from build123d import *

# Parameters (mm, degrees)
F0_R         = 8.5
F1_DEPTH     = 16
F2_DEPTH     = 4
F3_DEPTH     = 15
F4_W         = 9.6
F4_H         = 9.6
F5_DEPTH     = 11
F6_T1_DEPTH  = 10
F6_T3_DEPTH  = 7.6
F6_T5_DEPTH  = 7.6
F6_S9_W      = 1.02
F6_S9_H      = 1.02
F6_T10_DEPTH = 1.02
F6_S15_W     = 1.02
F6_S15_H     = 1.02
F6_T16_DEPTH = 1.02
F6_S21_W     = 1.02
F6_S21_H     = 1.02
F6_T22_DEPTH = 1.02
F6_S27_W     = 1.02
F6_S27_H     = 1.02
F6_T28_DEPTH = 1.02
F7_SIZE2     = 25
F7_SIZE      = 1
F8_T1_DEPTH  = 4
F8_T3_DEPTH  = 4
F9_DEPTH     = 25


# Not quite as in the source:
# - a fillet or chamfer that OpenCascade refuses, or shapes differently, is made with other operations: its cross-section is extruded or revolved along the edge and cut away or added


with BuildPart() as f1:
    # F0 (on Top) → F1 (new body)
    with BuildSketch(Plane.XY):
        Circle(F0_R)
        with BuildLine():
            Line((3.4119543857, 2.130107217), (3.5507041555, 2.05))
            Line((3.5507041555, 2.05), (3.5507041555, -2.05))
            Line((3.5507041555, -2.05), (3.4119543857, -2.130107217))
            ThreePointArc((3.4119543857, -2.130107217), (0, -4.85), (-3.4119543857, -2.130107217))
            Line((-3.4119543857, -2.130107217), (-3.5507041555, -2.05))
            Line((-3.5507041555, -2.05), (-3.5507041555, 2.05))
            Line((-3.5507041555, 2.05), (-3.4119543857, 2.130107217))
            ThreePointArc((-3.4119543857, 2.130107217), (0, 4.85), (3.4119543857, 2.130107217))
        make_face(mode=Mode.SUBTRACT)
    extrude(amount=F1_DEPTH)

    # F0 (on Top) → F2 (join)
    with BuildSketch(Plane.XY):
        with BuildLine():
            Line((0, 4.1), (3.4119543857, 2.130107217))
            ThreePointArc((3.4119543857, 2.130107217), (0, 4.85), (-3.4119543857, 2.130107217))
            Line((-3.4119543857, 2.130107217), (0, 4.1))
        make_face()
        with BuildLine():
            ThreePointArc((-3.4119543857, -2.130107217), (0, -4.85), (3.4119543857, -2.130107217))
            Line((3.4119543857, -2.130107217), (0, -4.1))
            Line((0, -4.1), (-3.4119543857, -2.130107217))
        make_face()
    extrude(amount=F2_DEPTH)

    # F0 (on Top) → F3 (join)
    with BuildSketch(Plane.XY):
        Circle(F0_R)
        with BuildLine():
            Line((3.4119543857, 2.130107217), (3.5507041555, 2.05))
            Line((3.5507041555, 2.05), (3.5507041555, -2.05))
            Line((3.5507041555, -2.05), (3.4119543857, -2.130107217))
            ThreePointArc((3.4119543857, -2.130107217), (0, -4.85), (-3.4119543857, -2.130107217))
            Line((-3.4119543857, -2.130107217), (-3.5507041555, -2.05))
            Line((-3.5507041555, -2.05), (-3.5507041555, 2.05))
            Line((-3.5507041555, 2.05), (-3.4119543857, 2.130107217))
            ThreePointArc((-3.4119543857, 2.130107217), (0, 4.85), (3.4119543857, 2.130107217))
        make_face(mode=Mode.SUBTRACT)
        with BuildLine():
            ThreePointArc((-3.5, 1.35), (-3.4779189431, 1.7425300307), (-3.4119543857, 2.130107217))
            Line((-3.4119543857, 2.130107217), (-3.5507041555, 2.05))
            Line((-3.5507041555, 2.05), (-3.5507041555, -2.05))
            Line((-3.5507041555, -2.05), (-3.4119543857, -2.130107217))
            ThreePointArc((-3.4119543857, -2.130107217), (-3.4779189431, -1.7425300307), (-3.5, -1.35))
            Line((-3.5, -1.35), (-3.5, 1.35))
        make_face()
        with BuildLine():
            Line((0, 4.1), (3.4119543857, 2.130107217))
            ThreePointArc((3.4119543857, 2.130107217), (0, 4.85), (-3.4119543857, 2.130107217))
            Line((-3.4119543857, 2.130107217), (0, 4.1))
        make_face()
        with BuildLine():
            ThreePointArc((-3.4119543857, -2.130107217), (0, -4.85), (3.4119543857, -2.130107217))
            Line((3.4119543857, -2.130107217), (0, -4.1))
            Line((0, -4.1), (-3.4119543857, -2.130107217))
        make_face()
        with BuildLine():
            Line((3.5507041555, -2.05), (3.5507041555, 2.05))
            Line((3.5507041555, 2.05), (3.4119543857, 2.130107217))
            ThreePointArc((3.4119543857, 2.130107217), (3.4779189431, 1.7425300307), (3.5, 1.35))
            Line((3.5, 1.35), (3.5, -1.35))
            ThreePointArc((3.5, -1.35), (3.4779189431, -1.7425300307), (3.4119543857, -2.130107217))
            Line((3.4119543857, -2.130107217), (3.5507041555, -2.05))
        make_face()
    extrude(amount=-F3_DEPTH)

    # F4 (on face) → F5 (cut)
    with BuildSketch(Plane(origin=(0, 0, -15), x_dir=(1, 0, 0), z_dir=(0, 0, -1))):
        Rectangle(F4_W, F4_H)
        with BuildLine():
            Line((-3.4119543857, 2.130107217), (0, 4.1))
            Line((0, 4.1), (3.4119543857, 2.130107217))
            ThreePointArc((3.4119543857, 2.130107217), (3.4779189431, 1.7425300307), (3.5, 1.35))
            Line((3.5, 1.35), (3.5, -1.35))
            ThreePointArc((3.5, -1.35), (3.4779189431, -1.7425300307), (3.4119543857, -2.130107217))
            Line((3.4119543857, -2.130107217), (0, -4.1))
            Line((0, -4.1), (-3.4119543857, -2.130107217))
            ThreePointArc((-3.4119543857, -2.130107217), (-3.4779189431, -1.7425300307), (-3.5, -1.35))
            Line((-3.5, -1.35), (-3.5, 1.35))
            ThreePointArc((-3.5, 1.35), (-3.4779189431, 1.7425300307), (-3.4119543857, 2.130107217))
        make_face(mode=Mode.SUBTRACT)
    extrude(amount=-F5_DEPTH, mode=Mode.SUBTRACT)

    # F6: fillet of radius 1 on 8 edges, made by hand

    # F6_s2 → F6_t1 (join)
    with BuildSketch(Plane.XY.offset(-15)):
        with BuildLine():
            ThreePointArc((-4.8, -3.8), (-4.5071067812, -4.5071067812), (-3.8, -4.8))
            Line((-3.8, -4.8), (-4.8, -4.8))
            Line((-4.8, -4.8), (-4.8, -3.8))
        make_face()
        with BuildLine():
            ThreePointArc((-4.8, 3.8), (-4.5071067812, 4.5071067812), (-3.8, 4.8))
            Line((-3.8, 4.8), (-4.8, 4.8))
            Line((-4.8, 4.8), (-4.8, 3.8))
        make_face()
        with BuildLine():
            ThreePointArc((3.8, -4.8), (4.5071067812, -4.5071067812), (4.8, -3.8))
            Line((4.8, -3.8), (4.8, -4.8))
            Line((4.8, -4.8), (3.8, -4.8))
        make_face()
        with BuildLine():
            ThreePointArc((4.8, 3.8), (4.5071067812, 4.5071067812), (3.8, 4.8))
            Line((3.8, 4.8), (4.8, 4.8))
            Line((4.8, 4.8), (4.8, 3.8))
        make_face()
    extrude(amount=F6_T1_DEPTH)

    # F6_s4 → F6_t3 (join)
    with BuildSketch(Plane.YZ.offset(-3.8)):
        with BuildLine():
            ThreePointArc((4.8, -5), (4.5071067812, -4.2928932188), (3.8, -4))
            Line((3.8, -4), (4.8, -4))
            Line((4.8, -4), (4.8, -5))
        make_face()
        with BuildLine():
            ThreePointArc((-4.8, -5), (-4.5071067812, -4.2928932188), (-3.8, -4))
            Line((-3.8, -4), (-4.8, -4))
            Line((-4.8, -4), (-4.8, -5))
        make_face()
    extrude(amount=F6_T3_DEPTH)

    # F6_s6 → F6_t5 (join)
    with BuildSketch(Plane.XZ.offset(-3.8)):
        with BuildLine():
            ThreePointArc((-4.8, -5), (-4.5071067812, -4.2928932188), (-3.8, -4))
            Line((-3.8, -4), (-4.8, -4))
            Line((-4.8, -4), (-4.8, -5))
        make_face()
        with BuildLine():
            ThreePointArc((4.8, -5), (4.5071067812, -4.2928932188), (3.8, -4))
            Line((3.8, -4), (4.8, -4))
            Line((4.8, -4), (4.8, -5))
        make_face()
    extrude(amount=F6_T5_DEPTH)


with BuildPart() as f6_tool8:
    # F6_s9 → F6_t10 (new body)
    with BuildSketch(Plane.XY.offset(-5)):
        with Locations((-4.31, -4.31)):
            Rectangle(F6_S9_W, F6_S9_H)
    extrude(amount=F6_T10_DEPTH)

    # F6_s11 → F6_t12 (revolve, cut)
    with BuildSketch(Plane(origin=(-3.8, -3.8, -5), x_dir=(0.7071067812, 0.7071067812, 0), z_dir=(0.7071067812, -0.7071067812, 0))):
        with BuildLine():
            ThreePointArc((0, -1), (1, 0), (0, 1))
            Line((0, 1), (0, -1))
        make_face()
    revolve(axis=Axis((-3.8, -3.8, -5), (0, 0, 1)), mode=Mode.SUBTRACT)


with BuildPart() as f1_1:
    add(f1.part)

    # F6_t7: union F6_tool8
    add(f6_tool8.part)


with BuildPart() as f6_tool14:
    # F6_s15 → F6_t16 (new body)
    with BuildSketch(Plane.XY.offset(-5)):
        with Locations((-4.31, 4.31)):
            Rectangle(F6_S15_W, F6_S15_H)
    extrude(amount=F6_T16_DEPTH)

    # F6_s17 → F6_t18 (revolve, cut)
    with BuildSketch(Plane(origin=(-3.8, 3.8, -5), x_dir=(0.7071067812, -0.7071067812, 0), z_dir=(-0.7071067812, -0.7071067812, 0))):
        with BuildLine():
            ThreePointArc((0, -1), (1, 0), (0, 1))
            Line((0, 1), (0, -1))
        make_face()
    revolve(axis=Axis((-3.8, 3.8, -5), (0, 0, 1)), mode=Mode.SUBTRACT)


with BuildPart() as f1_2:
    add(f1_1.part)

    # F6_t13: union F6_tool14
    add(f6_tool14.part)


with BuildPart() as f6_tool20:
    # F6_s21 → F6_t22 (new body)
    with BuildSketch(Plane.XY.offset(-5)):
        with Locations((4.31, -4.31)):
            Rectangle(F6_S21_W, F6_S21_H)
    extrude(amount=F6_T22_DEPTH)

    # F6_s23 → F6_t24 (revolve, cut)
    with BuildSketch(Plane(origin=(3.8, -3.8, -5), x_dir=(-0.7071067812, 0.7071067812, 0), z_dir=(0.7071067812, 0.7071067812, 0))):
        with BuildLine():
            ThreePointArc((0, -1), (1, 0), (0, 1))
            Line((0, 1), (0, -1))
        make_face()
    revolve(axis=Axis((3.8, -3.8, -5), (0, 0, 1)), mode=Mode.SUBTRACT)


with BuildPart() as f1_3:
    add(f1_2.part)

    # F6_t19: union F6_tool20
    add(f6_tool20.part)


with BuildPart() as f6_tool26:
    # F6_s27 → F6_t28 (new body)
    with BuildSketch(Plane.XY.offset(-5)):
        with Locations((4.31, 4.31)):
            Rectangle(F6_S27_W, F6_S27_H)
    extrude(amount=F6_T28_DEPTH)

    # F6_s29 → F6_t30 (revolve, cut)
    with BuildSketch(Plane(origin=(3.8, 3.8, -5), x_dir=(-0.7071067812, -0.7071067812, 0), z_dir=(-0.7071067812, 0.7071067812, 0))):
        with BuildLine():
            ThreePointArc((0, -1), (1, 0), (0, 1))
            Line((0, 1), (0, -1))
        make_face()
    revolve(axis=Axis((3.8, 3.8, -5), (0, 0, 1)), mode=Mode.SUBTRACT)


with BuildPart() as f1_4:
    add(f1_3.part)

    # F6_t25: union F6_tool26
    add(f6_tool26.part)

    # F7
    f7_edges = [f1_4.edges().sort_by_distance(p)[0] for p in [
        (-8.5, 0, 16),
    ]]
    f7_side = f1_4.faces().sort_by_distance((-8.259584, 0, 16))[0]
    chamfer(f7_edges, length=F7_SIZE, length2=F7_SIZE2, reference=f7_side)

    # F8: fillet of radius 5 on 4 edges, made by hand

    # F8_s2 → F8_t1 (join)
    with BuildSketch(Plane.XY):
        with BuildLine():
            ThreePointArc((2.5, -2.656624327), (0, -3.3264973081), (-2.5, -2.656624327))
            Line((-2.5, -2.656624327), (0, -4.1))
            Line((0, -4.1), (2.5, -2.656624327))
        make_face()
        with BuildLine():
            ThreePointArc((2.5, 2.656624327), (0, 3.3264973081), (-2.5, 2.656624327))
            Line((-2.5, 2.656624327), (0, 4.1))
            Line((0, 4.1), (2.5, 2.656624327))
        make_face()
    extrude(amount=F8_T1_DEPTH)

    # F8_s4 → F8_t3 (join)
    with BuildSketch(Plane.XY.offset(-4)):
        with BuildLine():
            ThreePointArc((2.5, -2.656624327), (0, -3.3264973081), (-2.5, -2.656624327))
            Line((-2.5, -2.656624327), (0, -4.1))
            Line((0, -4.1), (2.5, -2.656624327))
        make_face()
        with BuildLine():
            ThreePointArc((2.5, 2.656624327), (0, 3.3264973081), (-2.5, 2.656624327))
            Line((-2.5, 2.656624327), (0, 4.1))
            Line((0, 4.1), (2.5, 2.656624327))
        make_face()
    extrude(amount=F8_T3_DEPTH)

    # F9 (cut): faces of the model
    f9_faces = [f1_4.faces().sort_by_distance(p)[0] for p in [
        (3.5168739038, 0, 0),
        (-3.5168739038, 0, 0),
    ]]
    extrude(f9_faces, amount=-F9_DEPTH, mode=Mode.SUBTRACT)


solid = f1_4.part
Source: CAD feature listing. Evaluate the final solid. Frame: model axes, mm. A direction names the side the tool comes from. Coordinates: 2 decimals unless noted, no trailing zeros. Loops run counter-clockwise (first coordinate to the right, second up) from the corner with the lowest first, then second, coordinate; pieces in that order, holes last. Notation, with made-up numbers: (3.5, 57.25) - (49.5, 57.25) arc R15 ccw to (49.5, 72.25) - close; hole circle Ø3 at (45, -27). An arc over 180 degrees is marked (long way). Return JSON: item names as keys, results as strings.
Q1. Section D-D, the plane z = 11.5. Return loops of the section in (x, y), plus the area to 3 significant figures.
Results:
{"outline": "circle Ø15.36 at (0, 0); hole (-3.55, -2.05) - (-3.41, -2.13) arc R3.5 ccw to (3.41, -2.13) - (3.55, -2.05) - (3.55, 2.05) - (3.41, 2.13) arc R3.5 ccw to (-3.41, 2.13) - (-3.55, 2.05) - close", "area": "127 mm2"}
Q2. Material intervals for line 1 along X through (y, z) = (0.5, -10.5); line 2 along Y through (x, z) = (3.25, -14); line 3 along X through (y, z) = (-3, 12), sorted ascending.
Results:
{"line 1": "-8.49 to -4.8, 4.8 to 8.49", "line 2": "-7.85 to -4.8, 4.8 to 7.85", "line 3": "-7.05 to -3.09, 3.09 to 7.05"}
Q3. Mould query, pull axis Y, two halves, no side actions, for faces 4 (the flat face through (3.2, -3.2, 16)), 5 (the conical face through (-1.736, -7.817, 3.325)), 6 (the flat face through (0, -4, 4)). Classes: released by +Y, released by -Y, zero draft, split by the parting line, or undercut.
Results:
{"face 4": "zero draft", "face 5": "split by the parting line", "face 6": "undercut"}
Q4. Contact query for flat-ended pins moving along their axis: P1, Ø2, axis at x = -0.5, y = 3.5, coming from the +Z side; P2, Ø3, axis at x = 6, z = -10, coming from the -Y side; P3, Ø2, axis at x = -6.5, z = 4, coming from the -Y side; P4, Ø8.5, axis at y = 1.5, z = -10.5, coming from the +X side. Output: stop coordinate, or through.
Results:
{"P1": "z = 4", "P2": "y = -7.21", "P3": "y = -5.78", "P4": "x = 8.5"}
Q5. Section B-B, the plane z = -6. Return loops of the section in (x, y), plus the area to 3 significant figures.
Results:
{"outline": "circle Ø16.76 at (0, 0); hole (-4.8, -3.8) arc R1 ccw to (-3.8, -4.8) - (3.8, -4.8) arc R1 ccw to (4.8, -3.8) - (4.8, 3.8) arc R1 ccw to (3.8, 4.8) - (-3.8, 4.8) arc R1 ccw to (-4.8, 3.8) - close", "area": "129 mm2"}
Q6. Access query for faces 1 (the cylindrical face through (-0.053, 4.515, -4.301)), 2 (the cylindrical face through (0.037, -3.326, -0.056)), 3 (the flat face through (0, 4, 4)). Directions: +Z, -Z, +X, -X, +Y, -Y. A direction counts if a zero-diameter tool reaches every point of the face in a straight line with its end or side. Return the directions, or none.
Results:
{"face 1": "-Z", "face 2": "+Z, -Z", "face 3": "+Z"}
Q7. Section C-C, the plane x = 0. Return loops of the section in (y, z), plus the area to 3 significant figures.
Results:
{"outline": "(-8.5, -15) - (-4.8, -15) - (-4.8, -5) arc R1 cw to (-3.8, -4) - (-3.33, -4) - (-3.33, 4) - (-4.85, 4) - (-4.85, 16) - (-7.5, 16) - (-8.5, -9) - close; (3.33, -4) - (3.8, -4) arc R1 cw to (4.8, -5) - (4.8, -15) - (8.5, -15) - (8.5, -9) - (7.5, 16) - (4.85, 16) - (4.85, 4) - (3.33, 4) - close", "area": "227 mm2"}
Q8. Section A-A, the plane y = 0. Return loops of the section in (x, z).
Results:
{"outline": "(-8.5, -15) - (-4.8, -15) - (-4.8, -5) arc R1 cw to (-3.8, -4) - (-3.55, -4) - (-3.55, 16) - (-7.5, 16) - (-8.5, -9) - close; (3.55, -4) - (3.8, -4) arc R1 cw to (4.8, -5) - (4.8, -15) - (8.5, -15) - (8.5, -9) - (7.5, 16) - (3.55, 16) - close"}
